Part model, mm, in its own coordinate system. Face numbers are marked on the shaded views. A direction names the side the tool comes from. Coordinates: 2 decimals unless noted, no trailing zeros. Order: outer loops, then holes, each group sorted by start corner. A loop starts at its lowest first (then second) coordinate and runs counter-clockwise, first axis right, second up. Notation, with made-up numbers: M 28.5,-23 L 75.5,-23 A29 cw 75.5,10 Z; hole C -35,14 d11. An arc over 180 degrees is marked long. Answer in a Markdown table with one row per item. Add a question column.
from build123d import *

# Parameters (mm, degrees)
F_4_40_TAPPED_HOLE1_REACH  = 51.289
F_4_40_TAPPED_HOLE1_BORE_R = 1.1303


with BuildPart() as part:
    # Sketch → Shaft (revolve)
    with BuildSketch(Plane(origin=(0, 0, 0), x_dir=(0, 0, -1), z_dir=(1, 0, 0))):
        Polygon((0, 0), (0, 3.175), (31.242, 3.175), (31.242, 9.525), (44.45, 9.525), (44.45, 6.35), (33.782, 6.35), (33.782, 0), align=None)
    revolve(axis=Axis((0, 0, -33.782), (0, 0, 1)))

    # #4-40 Tapped Hole1 bore → #4-40 Tapped Hole1 (cut, up to next)
    with BuildSketch(Plane(origin=(0, 9.525, 0), x_dir=(1, 0, 0), z_dir=(0, 1, 0)), mode=Mode.PRIVATE) as f_4_40_tapped_hole1_sk1:
        with Locations((0, 36.449)):
            Circle(F_4_40_TAPPED_HOLE1_BORE_R)
    f_4_40_tapped_hole1_tool1 = extrude(f_4_40_tapped_hole1_sk1.sketch, amount=-F_4_40_TAPPED_HOLE1_REACH, mode=Mode.PRIVATE) & part.part
    # #4-40 Tapped Hole1 bore → #4-40 Tapped Hole1 (cut, up to next)
    with BuildSketch(Plane(origin=(0, 9.525, 0), x_dir=(1, 0, 0), z_dir=(0, 1, 0)), mode=Mode.PRIVATE) as f_4_40_tapped_hole1_sk2:
        with Locations((0, 41.783)):
            Circle(F_4_40_TAPPED_HOLE1_BORE_R)
    f_4_40_tapped_hole1_tool2 = extrude(f_4_40_tapped_hole1_sk2.sketch, amount=-F_4_40_TAPPED_HOLE1_REACH, mode=Mode.PRIVATE) & part.part
    add(f_4_40_tapped_hole1_tool1.solids().sort_by_distance((0, 9.525, -36.449))[0], mode=Mode.SUBTRACT)
    add(f_4_40_tapped_hole1_tool2.solids().sort_by_distance((0, 9.525, -41.783))[0], mode=Mode.SUBTRACT)


solid = part.part
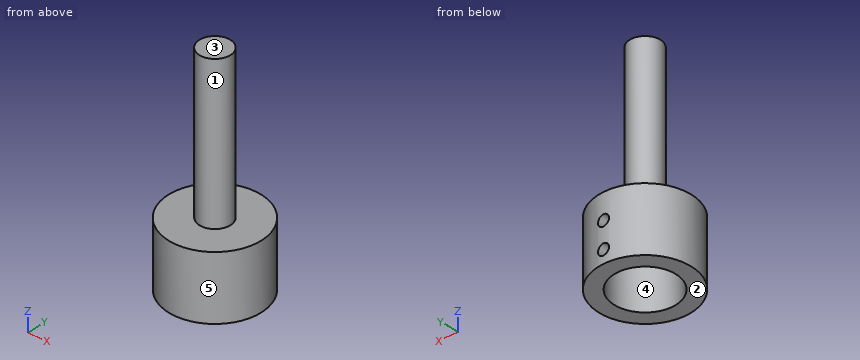
(1) Slice it at A-A (x = 0). List the corners of the cut face in (y, z) (3 decimals).
(2) Slice it at D-D (z = -4.5). List the corners of the cut face in (x, y) (3 decimals), and give its area (3 significant figures).
(3) Slice it at C-C (x = -5.25). List the corners of the cut face in (y, z), and give its area (3 significant figures).
(4) Slice it at B-B (y = 0). List the corners of the cut face in (x, z) (3 decimals).
(5) Drop flat-ended pins along their axis: P1, Ø10, axis at y = 4.5, z = -17, coming from the +X side (3 decimals); P2, Ø10, axis at y = -5.5, z = -9.5, coming from the -X side; P3, Ø10, axis at x = 5.5, z = -32.5, coming from the -Y side. Give the stop position or say it passes through.
(6) 3-axis set-ups, long thin cutter, end or side, ignore diameter. For the marked faces 1 and 2: which of +Z, -Z, +X, -X, +Y, -Y reach the whole face in a straight line?
(7) Wall check: line 1 (X direction, y = 0, z = -40.25) (3 decimals); line 2 (Z direction, x = 7, y = 6.25); line 3 (Z direction, x = -3.5, y = 3.75). Give the ranges that are in metal, low to high.
(8) Pull direction X, two halves, no side cores. Call the marked faces 3, 4 and 5: pulls with the +X half, pulls with the -X half, needs draft (parallel to the pull), parting line crosses it, or undercut.
Computed:
| question | item | result |
|---|---|---|
| 1 | outline | M -9.525,-44.45 L -6.35,-44.45 L -6.35,-33.782 L 6.35,-33.782 L 6.35,-35.319 L 9.525,-35.319 L 9.525,-31.242 L 3.175,-31.242 L 3.175,0 L -3.175,0 L -3.175,-31.242 L -9.525,-31.242 Z; M 6.35,-44.45 L 9.525,-44.45 L 9.525,-42.913 L 6.35,-42.913 Z; M 6.35,-40.653 L 9.525,-40.653 L 9.525,-37.579 L 6.35,-37.579 Z |
| 2 | outline | C 0,0 d6.35 |
| 2 | area | 31.7 mm^2 |
| 3 | outline | M -7.95,-44.45 L -3.57,-44.45 L -3.57,-33.78 L 3.57,-33.78 L 3.57,-44.45 L 7.95,-44.45 L 7.95,-31.24 L -7.95,-31.24 Z |
| 3 | area | 134 mm^2 |
| 4 | outline | M -9.525,-44.45 L -6.35,-44.45 L -6.35,-33.782 L 6.35,-33.782 L 6.35,-44.45 L 9.525,-44.45 L 9.525,-31.242 L 3.175,-31.242 L 3.175,0 L -3.175,0 L -3.175,-31.242 L -9.525,-31.242 Z |
| 5 | P1 | stops at x = 3.175 |
| 5 | P2 | stops at x = -3.14 |
| 5 | P3 | stops at y = -9.51 |
| 6 | face 1 | +Z |
| 6 | face 2 | -Z, +X, -X, +Y, -Y |
| 7 | line 1 | x = -9.525 to -6.35, 6.35 to 9.525 |
| 7 | line 2 | z = -44.45 to -31.24 |
| 7 | line 3 | z = -33.78 to -31.24 |
| 8 | face 3 | needs draft |
| 8 | face 4 | undercut |
| 8 | face 5 | parting line crosses it |
